Model file for the job. Use its own axes, mm. A direction names the side the tool comes from. Round coordinates to 2 decimals unless told otherwise and drop trailing zeros. Order: outer loops, then holes, each group sorted by start corner. A loop starts at its lowest first (then second) coordinate and runs counter-clockwise, first axis right, second up. Notation, with made-up numbers: (74.5, -38.5) - (81.5, -38.5) arc R22 cw to (81.5, -29.5) - close; hole circle Ø6 at (61.5, 47). An arc over 180 degrees is marked (long way). Write item = value, one per line.
```python
from build123d import *

# Parameters (mm, degrees)
F0_W     = 101.6
F0_H     = 101.6
F1_DEPTH = 50.8
F2_R     = 4.7348864271
F3_DEPTH = 101.601
F5_COUNT = 12
F5_ANGLE = 330
F6_W     = 50.8
F6_H     = 50.8
F7_DEPTH = 76.2


with BuildPart() as f1:
    # F0 (on Front) → F1 (new body, symmetric)
    with BuildSketch(Plane.XZ):
        Rectangle(F0_W, F0_H)
    extrude(amount=F1_DEPTH, both=True)

    # F2 (on face) → F3 (cut, through all)
    with BuildSketch(Plane.XZ.offset(50.8)):
        with Locations((-27.4963065702, 15.875)):
            Circle(F2_R)
    f3 = extrude(amount=-F3_DEPTH, mode=Mode.SUBTRACT)

    # F5: F3 ×12 about axis
    f5_axis = Axis((0, 0, 0), (0, -1, 0))
    for i in range(1, F5_COUNT):
        add(f3.rotate(f5_axis, i * F5_ANGLE / (F5_COUNT - 1)), mode=Mode.SUBTRACT)

    # F6 (on face) → F7 (cut)
    with BuildSketch(Plane.YZ.offset(50.8)):
        Rectangle(F6_W, F6_H)
    extrude(amount=-F7_DEPTH, mode=Mode.SUBTRACT)


solid = f1.part
```
1) Cut at B-B (x = 42). Write the cut outline in (y, z), and give its area (3 significant figures).
Conclusion:
outline = (-50.8, -50.8) - (50.8, -50.8) - (50.8, 50.8) - (-50.8, 50.8) - close; hole (-25.4, -25.4) - (25.4, -25.4) - (25.4, 25.4) - (-25.4, 25.4) - close
area = 7,740 mm^2
2) Flat gauge pin, fed straight in: pin 1 Ø11.5 at (y, z) = (-9, -5.5) entering from +X. Where does the tip first touch, or does it go through?
Conclusion:
pin_1 = -25.4
3) Cut at D-D (z = -18). Write the cut outline in (x, y).
Conclusion:
outline = (-50.8, -50.8) - (-31.73, -50.8) - (-31.73, 50.8) - (-50.8, 50.8) - close; (-23.27, -50.8) - (23.27, -50.8) - (23.27, -25.4) - (-23.27, -25.4) - close; (-23.27, 25.4) - (23.27, 25.4) - (23.27, 50.8) - (-23.27, 50.8) - close; (31.73, -50.8) - (50.8, -50.8) - (50.8, -25.4) - (31.73, -25.4) - close; (31.73, 25.4) - (50.8, 25.4) - (50.8, 50.8) - (31.73, 50.8) - close
4) Wall check: line 1 along Y through (x, z) = (11.5, -11.5); line 2 along X through (y, z) = (28, 11.5). Give the ranges that are in metal, low to high.
Conclusion:
line_1 = -50.8 to -25.4, 25.4 to 50.8
line_2 = -50.8 to -29.31, -25.69 to 25.69, 29.31 to 50.8
5) Cut at A-A (x = 0). Write the cut outline in (y, z), and give its area (3 significant figures).
Conclusion:
outline = (-50.8, -50.8) - (50.8, -50.8) - (50.8, -36.48) - (-50.8, -36.48) - close; (-50.8, -27.02) - (50.8, -27.02) - (50.8, 27.02) - (-50.8, 27.02) - close; (-50.8, 36.48) - (50.8, 36.48) - (50.8, 50.8) - (-50.8, 50.8) - close; hole (-25.4, -25.4) - (25.4, -25.4) - (25.4, 25.4) - (-25.4, 25.4) - close
area = 5,820 mm^2
6) Mould opens along Y. For faces 3 (the face through (-25.4, 0, -23)), 4 (the face through (-1, 50.8, 1)), 5 (the face through (32.227, 37.922, -16.083)) say: +Y half, -Y half, draft (parallel to the pull), parting line (faces both ways), or undercut.
Conclusion:
face_3 = undercut
face_4 = +Y half
face_5 = draft
7) Cut at C-C (y = -39). Give the number of separate pieces and of enclosed holes in the cut face, and give its area (3 significant figures).
Conclusion:
separate_pieces = 1
enclosed_holes = 12
area = 9,480 mm^2
8) 3-axis set-ups, long thin cutter, end or side, ignore diameter. For faces 1 (the face through (-25.4, 0, 0)), 2 (the face through (-1, -1, -50.8)): which of +Z, -Z, +X, -X, +Y, -Y reach the whole face in a straight line?
Conclusion:
face_1 = +X
face_2 = -Z, +X, -X, +Y, -Y
